Geometry: final body of the model. Coordinates: model frame, mm. A direction names the side the tool comes from. Give positions to 0.01 mm unless a question says otherwise; leave off trailing zeros. Order: outer loops, then holes, each group sorted by start corner. A loop starts at its lowest first (then second) coordinate and runs counter-clockwise, first axis right, second up. Notation, with made-up numbers: (60, 87) -> (71, 87) arc R16 ccw to (71, 113) -> close; hole circle Ø1 at (-33.5, 31.25). An arc over 180 degrees is marked (long way). Answer in a Markdown table with one row per item. Add a question column.
Q1. Pull-direction query (Z, two-part tool) for faces 1 (the face through (-30.398, 73.042, -31.086)), 2 (the face through (8, 76, -1)), 3 (the face through (1.76, 34.51, -39.96)); classes: +Z half, -Z half, draft (parallel to the pull), parting line (faces both ways), or undercut.
Q2. Cut plane B-B on z = -13. Return the cut outline in (x, y), and give its area (3 significant figures).
Q3. Set-up query: faces 4 (the face through (1, 71, 3)), 5 (the face through (0, 24.166, 37)), 6 (the face through (1, 0, -1)). Return all of +Z, -Z, +X, -X, +Y, -Y with unobstructed straight access to the full face (end or side cutting, diameter ignored); none if empty.
Q4. Line query: line 1 along X through (y, z) = (75.5, 0); line 2 along X through (y, z) = (73.7, 0); line 3 along Y through (x, z) = (-0.5, 20). Output: solid intervals per line, ascending. Write a range as from..to.
Q5. Cut plane A-A on x = 0. Return the cut outline in (y, z), and give its area (3 significant figures).
Q6. Cut plane D-D on x = -18.5. Return the cut outline in (y, z).
Q7. Contact query for flat-ended pins moving along their axis: P1, Ø2, axis at x = 30, z = -14.5, coming from the -Y side; P2, Ø12, axis at y = 18, z = 7, coming from the -X side; P3, Ø24, axis at x = 16, z = 16.5, coming from the +Y side; P4, Ø2.5, axis at x = -32.3, z = 32.3, coming from the +Y side (3 decimals). Output: stop coordinate, or through.
Q8. Cut plane C-C on y = 88. Return the cut outline in (x, z).
from build123d import *

# Parameters (mm, degrees)
SKETCH1_R                 = 40
BOSS_EXTRUDE1_DEPTH       = 70
SKETCH2_W                 = 95
SKETCH2_H                 = 95
BOSS_EXTRUDE2_DEPTH       = 6
SKETCH3_R                 = 40
SKETCH3_R_2               = 38.709273032
CUT_EXTRUDE1_DEPTH        = 1
SKETCH4_R                 = 3
BOSS_EXTRUDE3_DEPTH       = 61
FILLET1_R                 = 8
SKETCH6_R                 = 3.519560707
SKETCH6_R_2               = 3
CUT_EXTRUDE3_DEPTH        = 5
CUT_EXTRUDE4_REACH        = 158.583
CUT_EXTRUDE4_START_RADIUS = 40
CUT_EXTRUDE4_END_RADIUS   = 40
SKETCH8_W                 = 29.147137568
SKETCH8_H                 = 8.22098752
BOSS_EXTRUDE5_DEPTH       = 4
SKETCH10_R                = 2.25
CUT_EXTRUDE5_DEPTH        = 34


with BuildPart() as part:
    # Sketch1 → Boss-Extrude1 (new body)
    with BuildSketch(Plane(origin=(0, 0, 0), x_dir=(1, 0, 0), z_dir=(0, 1, 0))):
        with Locations(Location((0, 0, 0), (0, 0, 270))):
            Circle(SKETCH1_R)
    extrude(amount=BOSS_EXTRUDE1_DEPTH)

    # Sketch2 → Boss-Extrude2 (add)
    with BuildSketch(Plane(origin=(0, 70, 0), x_dir=(1, 0, 0), z_dir=(0, 1, 0))):
        Rectangle(SKETCH2_W, SKETCH2_H)
    extrude(amount=BOSS_EXTRUDE2_DEPTH)

    # Sketch3 → Cut-Extrude1 (cut)
    with BuildSketch(Plane(origin=(0, 76, 0), x_dir=(1, 0, 0), z_dir=(0, 1, 0))):
        with Locations(Location((0, 0, 0), (0, 0, 270))):
            Circle(SKETCH3_R)
        with Locations(Location((0, 0, 0), (0, 0, 270))):
            Circle(SKETCH3_R_2, mode=Mode.SUBTRACT)
    extrude(amount=-CUT_EXTRUDE1_DEPTH, mode=Mode.SUBTRACT)

    # Sketch4 → Boss-Extrude3 (add)
    with BuildSketch(Plane(origin=(0, 76, 0), x_dir=(1, 0, 0), z_dir=(0, 1, 0))):
        with Locations(Location((0, 0, 0), (0, 0, 90))):
            Circle(SKETCH4_R)
    extrude(amount=BOSS_EXTRUDE3_DEPTH)

    # Fillet1
    fillet1_edges = [part.edges().sort_by_distance(p)[0] for p in [
        (47.5, 73, 47.5),
        (47.5, 73, -47.5),
        (-47.5, 73, -47.5),
        (-47.5, 73, 47.5),
    ]]
    fillet(fillet1_edges, radius=FILLET1_R)

    # Sketch6 → Cut-Extrude3 (cut)
    with BuildSketch(Plane(origin=(0, 76, 0), x_dir=(1, 0, 0), z_dir=(0, 1, 0))):
        with Locations(Location((0, 0, 0), (0, 0, 270))):
            Circle(SKETCH6_R)
        with Locations(Location((0, 0, 0), (0, 0, 90))):
            Circle(SKETCH6_R_2, mode=Mode.SUBTRACT)
    extrude(amount=-CUT_EXTRUDE3_DEPTH, mode=Mode.SUBTRACT)

    # Cut-Extrude4: from a cylinder face, 158.583 long prism both ways, kept between that surface and its translate by the depth
    cut_extrude4_start = Plane(origin=(0, 20.055809, 0), z_dir=(0, -1, 0)) * Cylinder(CUT_EXTRUDE4_START_RADIUS, 398.166, mode=Mode.PRIVATE)
    cut_extrude4_end = Plane(origin=(0, 20.055809, -4), z_dir=(0, -1, 0)) * Cylinder(CUT_EXTRUDE4_END_RADIUS, 398.166, mode=Mode.PRIVATE)
    # Sketch8 → Cut-Extrude4 (cut, from a surface)
    with BuildSketch(Plane.XY, mode=Mode.PRIVATE) as cut_extrude4_sk1:
        with Locations((0, 20.055809212)):
            Rectangle(SKETCH8_W, SKETCH8_H)
    cut_extrude4_tool1 = extrude(cut_extrude4_sk1.sketch, amount=CUT_EXTRUDE4_REACH, both=True, mode=Mode.PRIVATE)
    add(((cut_extrude4_tool1 & cut_extrude4_start) - cut_extrude4_end).solids().sort_by_distance((0, 20.055809, 35.250652))[0], mode=Mode.SUBTRACT)

    # Sketch9 → Boss-Extrude5 (add)
    with BuildSketch(Plane.XZ):
        with BuildLine():
            ThreePointArc((-25.622676251, -4.384366141), (-27.880429407, -0.093420807), (-25.772900348, 4.273269294))
            Line((-25.772900348, 4.273269294), (-27.319093183, 6.289872554))
            ThreePointArc((-27.319093183, 6.289872554), (-29.604344551, 3.506882349), (-30.422381519, 0))
            ThreePointArc((-30.422381519, 0), (-29.542433802, -3.629669529), (-27.097976665, -6.453397238))
            Line((-27.097976665, -6.453397238), (-25.622676251, -4.384366141))
        make_face()
    boss_extrude5 = extrude(amount=BOSS_EXTRUDE5_DEPTH)

    # Mirror1: Boss-Extrude5 across plane
    add(boss_extrude5.mirror(Plane(origin=(0, 0, 0), x_dir=(0, 0, 1), z_dir=(1, 0, 0))))

    # Sketch10 → Cut-Extrude5 (cut)
    with BuildSketch(Plane(origin=(0, 76, 0), x_dir=(1, 0, 0), z_dir=(0, 1, 0))):
        with Locations(Location((-32.295599691, 32.295599691, 0), (0, 0, 270))):
            Circle(SKETCH10_R)
        with Locations(Location((32.295599691, 32.295599691, 0), (0, 0, 270))):
            Circle(SKETCH10_R)
        with Locations(Location((32.295599691, -32.295599691, 0), (0, 0, 270))):
            Circle(SKETCH10_R)
        with Locations(Location((-32.295599691, -32.295599691, 0), (0, 0, 270))):
            Circle(SKETCH10_R)
    extrude(amount=-CUT_EXTRUDE5_DEPTH, mode=Mode.SUBTRACT)


solid = part.part
Completed:
| question | item | result |
|---|---|---|
| 1 | face 1 | undercut |
| 1 | face 2 | draft |
| 1 | face 3 | parting line |
| 2 | outline | (-47.5, 70) -> (-37.83, 70) -> (-37.83, 0) -> (37.83, 0) -> (37.83, 70) -> (47.5, 70) -> (47.5, 76) -> (37.83, 76) -> (37.83, 75) -> (36.46, 75) -> (36.46, 76) -> (-36.46, 76) -> (-36.46, 75) -> (-37.83, 75) -> (-37.83, 76) -> (-47.5, 76) -> close |
| 2 | area | 5,860 mm² |
| 3 | face 4 | +Y |
| 3 | face 5 | +Z |
| 3 | face 6 | -Y |
| 4 | line 1 | x = -47.5..-40, -38.71..-3.52, -3..3, 3.52..38.71, 40..47.5 |
| 4 | line 2 | x = -47.5..-3.52, -3..3, 3.52..47.5 |
| 4 | line 3 | y = 0..76 |
| 5 | outline | (0, -40) -> (70, -40) -> (70, -47.5) -> (76, -47.5) -> (76, -40) -> (75, -40) -> (75, -38.71) -> (76, -38.71) -> (76, -3.52) -> (71, -3.52) -> (71, -3) -> (137, -3) -> (137, 3) -> (71, 3) -> (71, 3.52) -> (76, 3.52) -> (76, 38.71) -> (75, 38.71) -> (75, 40) -> (76, 40) -> (76, 47.5) -> (70, 47.5) -> (70, 40) -> (24.17, 40) -> (24.17, 36) -> (15.95, 36) -> (15.95, 40) -> (0, 40) -> close |
| 5 | area | 6,500 mm² |
| 6 | outline | (0, -35.46) -> (70, -35.46) -> (70, -47.5) -> (76, -47.5) -> (76, -35.46) -> (75, -35.46) -> (75, -34) -> (76, -34) -> (76, 34) -> (75, 34) -> (75, 35.46) -> (76, 35.46) -> (76, 47.5) -> (70, 47.5) -> (70, 35.46) -> (0, 35.46) -> close |
| 7 | P1 | stops at y = 0 |
| 7 | P2 | stops at x = -39.99 |
| 7 | P3 | stops at y = 76 |
| 7 | P4 | passes through |
| 8 | outline | circle Ø6 at (0, 0) |
